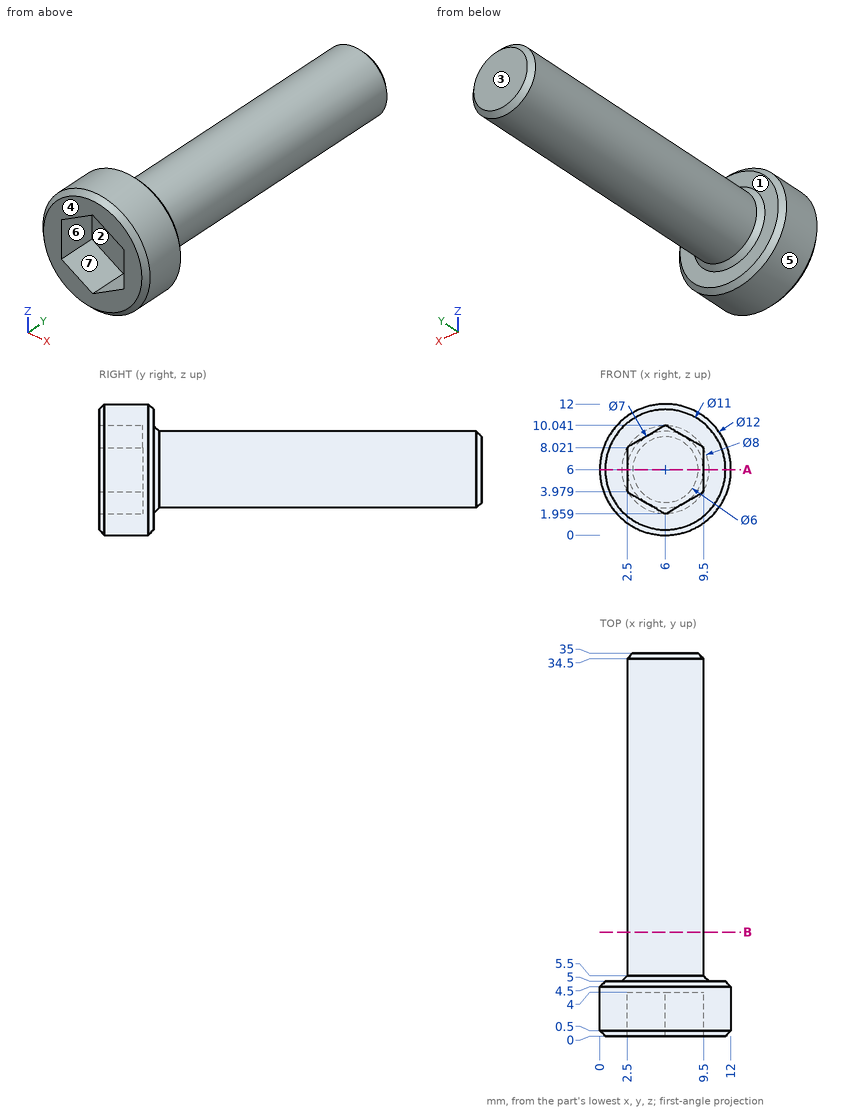
The drawing under review shows one solid part. Ordinate dimensions are in mm from its lowest x, y, z. A direction names the side the tool comes from. Round coordinates to 2 decimals unless told otherwise and drop trailing zeros. Order: outer loops, then holes, each group sorted by start corner. A loop starts at its lowest first (then second) coordinate and runs counter-clockwise, first axis right, second up. Notation, with made-up numbers: M 57.25,71.25 L 107.25,71.25 A19 cw 107.25,80.25 Z; hole C 46,56.5 d10. An arc over 180 degrees is marked long. Answer as CSV lines item,"result". Start each with the question number.
1) Tool access review of the marked faces 1, 2 and 3: name each direction out of +Z, -Z, +X, -X, +Y, -Y from which nothing blocks a thin tool from reaching the whole face with its end or side.
2) Add section A-A (z = 6). Give the boundary of the cut face in (x, y).
3) For pin 1 Ø6 at (x, y) = (1.5, 29) entering from +Z; pin 2 Ø2 at (x, y) = (2, 29.5) entering from -Z (1 decimal); pin 3 Ø2 at (x, y) = (9.5, 31.5) entering from +Z, all flat-tipped, find the tip position at first contact; note any pin that passes through.
4) The part is to be moulded in two halves that separate along X. For the marked faces 4, 5, 6 and 7, say which applies: +X half, -X half, draft (parallel to the pull), parting line (faces both ways), or undercut.
5) Add section B-B (y = 9.5). Give the boundary of the cut face in (x, z).
6) Wall thickness on line 1 along Y through (x, z) = (10.75, 6.25); line 2 along X through (y, z) = (2, 8.5) (1 decimal); line 3 along Y through (x, z) = (8.75, 5): over which ranges is each line inside the solid? List them lowest first. Write a range as [from, to].
Resolved:
1,face 1,"+Y"
1,face 2,"-Y"
1,face 3,"+Z, -Z, +X, -X, +Y"
2,outline,"M 0,0.5 L 0.5,0 L 2.5,0 L 2.5,4 L 9.5,4 L 9.5,0 L 11.5,0 L 12,0.5 L 12,4.5 L 11.5,5 L 10,5 L 9.5,5.5 L 9.5,34.5 L 9,35 L 3,35 L 2.5,34.5 L 2.5,5.5 L 2,5 L 0.5,5 L 0,4.5 Z"
3,pin 1,"z = 9.16"
3,pin 2,"z = 4.2"
3,pin 3,"z = 8.45"
4,face 4,"draft"
4,face 5,"parting line"
4,face 6,"undercut"
4,face 7,"undercut"
5,outline,"C 6,6 d7"
6,line 1,"[0, 5]"
6,line 2,"[0.5, 3.3], [8.7, 11.5]"
6,line 3,"[4, 35]"
